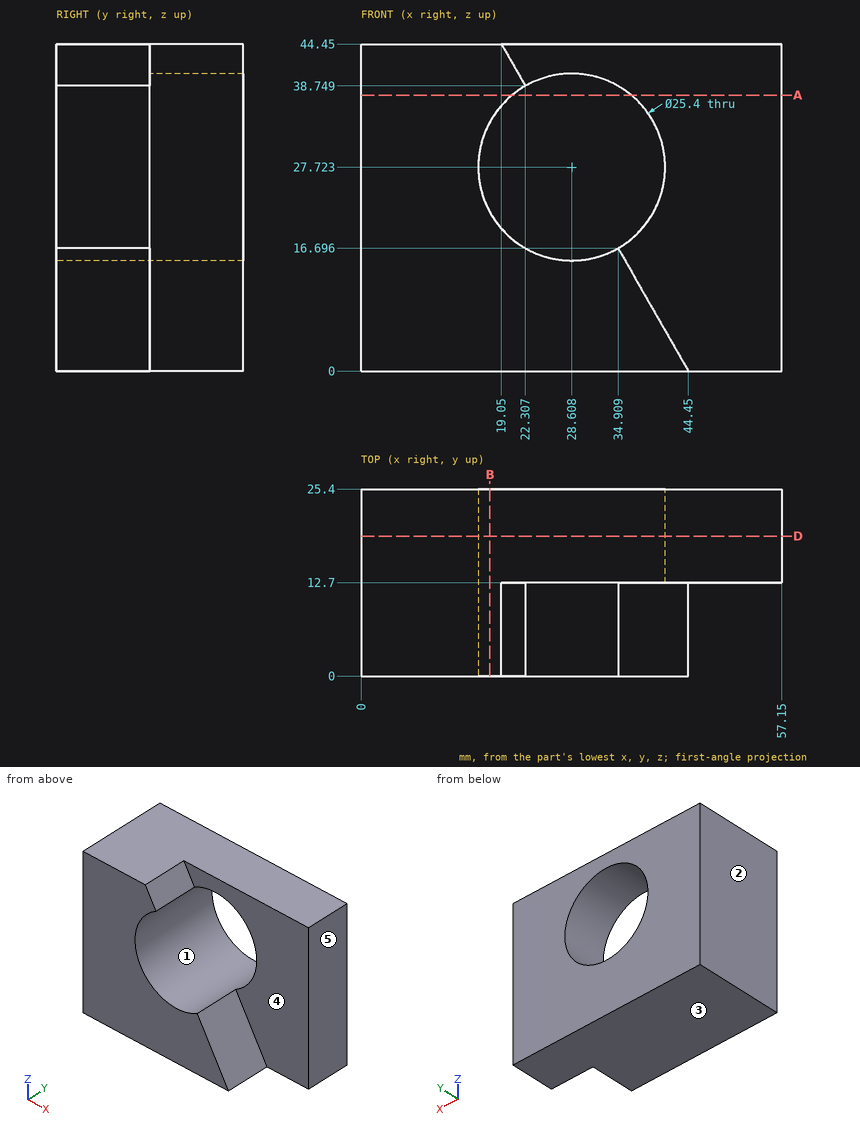
Source: three-view drawing plus pictorial views. Frame: mm from the lowest corner of the part. A direction names the side the tool comes from. Coordinates: 2 decimals unless noted, no trailing zeros. Write each loop counter-clockwise with the first axis right and the second up, starting at its lowest first coordinate (ties: lowest second). Pieces come first, ordered by that corner, then holes. Notation, with made-up numbers: (3, -14.75) -> (14, -14.75) arc R36 cw to (14, 19.25) -> close; hole circle Ø2 at (73, 83.25). An arc over 180 degrees is marked (long way). Answer as a JSON object with one key per item and string values.
1. Section B-B on x = 17.5. Return the cut outline in (y, z).
Result set:
{"outline": "(0, 0) -> (25.4, 0) -> (25.4, 21.57) -> (0, 21.57) -> close; (0, 33.88) -> (25.4, 33.88) -> (25.4, 44.45) -> (0, 44.45) -> close"}
2. Section A-A on z = 37.5. Return the cut outline in (x, y).
Result set:
{"outline": "(0, 0) -> (20.5, 0) -> (20.5, 25.4) -> (0, 25.4) -> close; (36.71, 12.7) -> (57.15, 12.7) -> (57.15, 25.4) -> (36.71, 25.4) -> close"}
3. First-contact query: P1, Ø23, axis at x = 28.61, z = 27.72, coming from the +Y side; P2, Ø1, axis at x = 41.5, z = 8, coming from the -Y side; P3, Ø8, axis at y = 4, z = 5, coming from the +X side; P4, Ø2, axis at y = 9.5, z = 25, coming from the +X side. Flat tips, straight axial feed; report the tip coordinate or a pass-through.
Result set:
{"P1": "passes through", "P2": "stops at y = 12.7", "P3": "stops at x = 43.88", "P4": "stops at x = 16.47"}
4. Material intervals for line 1 (Y direction, x = 51, z = 13.5); line 2 (X direction, y = 16, z = 29.5); line 3 (X direction, y = 12.5, z = 16) (1 decimal), sorted ascending. Write a range as from..to.
Result set:
{"line 1": "y = 12.7..25.4", "line 2": "x = 0..16.03, 41.18..57.15", "line 3": "x = 0..23.7, 33.5..35.3"}
5. Access query for the marked faces 4 and 5. Directions: +Z, -Z, +X, -X, +Y, -Y. A direction counts if a zero-diameter tool reaches every point of the face in a straight line with its end or side. Return the directions, or none.
Result set:
{"face 4": "+Z, +X, -Y", "face 5": "+Z, -Z, +X, +Y, -Y"}
6. Mould query, pull axis Z, two halves, no side actions, for the marked faces 1, 2 and 3. Classes: released by +Z, released by -Z, zero draft, split by the parting line, or undercut.
Result set:
{"face 1": "undercut", "face 2": "zero draft", "face 3": "released by -Z"}
7. Section D-D on y = 19. Return the cut outline in (x, z), then the cut area to 3 significant figures.
Result set:
{"outline": "(0, 0) -> (57.15, 0) -> (57.15, 44.45) -> (0, 44.45) -> close; hole circle Ø25.4 at (28.61, 27.72)", "area": "2,030 mm2"}
